Verification items for the finished model (mm, model axes). Round coordinates to 2 decimals unless told otherwise and drop trailing zeros. Write each loop counter-clockwise with the first axis right and the second up, starting at its lowest first coordinate (ties: lowest second). Pieces come first, ordered by that corner, then holes. Notation, with made-up numbers: (3.5, 14.25) - (7.5, 14.25) arc R26 cw to (7.5, 31.25) - close; hole circle Ø5 at (8, 5). An arc over 180 degrees is marked (long way). Answer as a JSON object with one key per item and string values. Group by question number.
1) Section check B-B (z = 143). Enter the section's corners in (x, y).
2) Section check D-D (x = -1). State how many separate pieces and enclosed holes the cut face has, then the cut area to 3 significant figures.
3) Go/stop test with flat-tipped pins: pin 1 Ø4 at (x, z) = (-5.5, 96) entering from -Y; pin 2 Ø6 at (x, y) = (-3, -152) entering from +Z. Record where each tip stops, or that it passes through.
4) Section check C-C (y = -149). Enter the section's corners in (x, z).
5) Thickness scan on line 1 (Z direction, x = 3.5, y = 904); line 2 (Y direction, x = -4.25, z = 289.5); line 3 (Z direction, x = 9, y = 1010). Record the ranges inside material, lowest first.
6) Section check A-A (y = 163). Enter the section's corners in (x, z).
```python
from build123d import *

# Parameters (mm, degrees)
SKETCH1_W           = 2
SKETCH1_H           = 2
SKETCH1_W_2         = 1.6
SKETCH1_H_2         = 1.6
BOSS_EXTRUDE1_DEPTH = 109
SKETCH2_W           = 2
SKETCH2_H           = 2
SKETCH2_W_2         = 1.6
SKETCH2_H_2         = 1.6
BOSS_EXTRUDE2_DEPTH = 34
SKETCH3_W           = 2
SKETCH3_H           = 2
SKETCH3_W_2         = 1.6
SKETCH3_H_2         = 1.6
BOSS_EXTRUDE3_DEPTH = 6
SKETCH7_W           = 2
SKETCH7_H           = 2
SKETCH7_W_2         = 1.54
SKETCH7_H_2         = 1.54
BOSS_EXTRUDE4_DEPTH = 36
BOSS_EXTRUDE5_REACH = 28
SKETCH8_W           = 2
SKETCH8_H           = 2
SKETCH8_W_2         = 1.6
SKETCH8_H_2         = 1.6
SCALE2_SCALE        = 10
BOSS_EXTRUDE6_REACH = 1412
SKETCH9_W           = 20
SKETCH9_H           = 20
SKETCH9_W_2         = 16
SKETCH9_H_2         = 16
SKETCH10_W          = 20
SKETCH10_H          = 20
SKETCH10_W_2        = 16
SKETCH10_H_2        = 16
BOSS_EXTRUDE7_DEPTH = 179.85


with BuildPart() as part:
    # Sketch1 → Boss-Extrude1 (new body)
    with BuildSketch(Plane(origin=(0, 0, 0), x_dir=(1, 0, 0), z_dir=(0, 1, 0))):
        Rectangle(SKETCH1_W, SKETCH1_H)
        Rectangle(SKETCH1_W_2, SKETCH1_H_2, mode=Mode.SUBTRACT)
    boss_extrude1 = extrude(amount=BOSS_EXTRUDE1_DEPTH)

    # Sketch2 → Boss-Extrude2 (add)
    with BuildSketch(Plane.XY.offset(1)):
        with Locations((0, 108)):
            Rectangle(SKETCH2_W, SKETCH2_H)
        with Locations((0, 108)):
            Rectangle(SKETCH2_W_2, SKETCH2_H_2, mode=Mode.SUBTRACT)
    extrude(amount=BOSS_EXTRUDE2_DEPTH)

    # Mirror1: Boss-Extrude1 across plane
    add(boss_extrude1.mirror(Plane.XY.offset(17)))

    # Sketch3 → Boss-Extrude3 (add)
    with BuildSketch(Plane.XY.offset(1)):
        with Locations((0, 1)):
            Rectangle(SKETCH3_W, SKETCH3_H)
        with Locations((0, 1)):
            Rectangle(SKETCH3_W_2, SKETCH3_H_2, mode=Mode.SUBTRACT)
    boss_extrude3 = extrude(amount=BOSS_EXTRUDE3_DEPTH)

    # Sketch7 → Boss-Extrude4 (add)
    with BuildSketch(Plane(origin=(0, 2, 0), x_dir=(1, 0, 0), z_dir=(0, 1, 0))):
        with Locations((0, -8)):
            Rectangle(SKETCH7_W, SKETCH7_H)
        with Locations((0, -8)):
            Rectangle(SKETCH7_W_2, SKETCH7_H_2, mode=Mode.SUBTRACT)
    boss_extrude4 = extrude(amount=-BOSS_EXTRUDE4_DEPTH)

    # Mirror2: Boss-Extrude3, Boss-Extrude4 across plane
    add(boss_extrude3.mirror(Plane.XY.offset(17)))
    add(boss_extrude4.mirror(Plane.XY.offset(17)))

    # Sketch8 → Boss-Extrude5 (add, up to next)
    with BuildSketch(Plane(origin=(0, 0, 25), x_dir=(-1, 0, 0), z_dir=(0, 0, -1)), mode=Mode.PRIVATE) as boss_extrude5_sk1:
        with Locations((0, -33)):
            Rectangle(SKETCH8_W, SKETCH8_H)
        with Locations((0, -33)):
            Rectangle(SKETCH8_W_2, SKETCH8_H_2, mode=Mode.SUBTRACT)
    boss_extrude5_tool1 = extrude(boss_extrude5_sk1.sketch, amount=BOSS_EXTRUDE5_REACH, mode=Mode.PRIVATE) - part.part
    add(boss_extrude5_tool1.solids().sort_by_distance((0, -32.028284, 25))[0])


with BuildPart() as part_1:
    # Scale2: scaled about (0, 0, 0)
    add(part.part.scale(SCALE2_SCALE))

    # Sketch9 → Boss-Extrude6 (add, up to next)
    with BuildSketch(Plane.XZ.offset(-1070), mode=Mode.PRIVATE) as boss_extrude6_sk1:
        with Locations((0, 169.738105544)):
            Rectangle(SKETCH9_W, SKETCH9_H)
        with Locations((0, 169.738105544)):
            Rectangle(SKETCH9_W_2, SKETCH9_H_2, mode=Mode.SUBTRACT)
    boss_extrude6_tool1 = extrude(boss_extrude6_sk1.sketch, amount=BOSS_EXTRUDE6_REACH, mode=Mode.PRIVATE) - part_1.part
    add(boss_extrude6_tool1.solids().sort_by_distance((0, 1070, 179.455263))[0])

    # Sketch10 → Boss-Extrude7 (add)
    with BuildSketch(Plane.XZ.offset(340)):
        with Locations((0, 170)):
            Rectangle(SKETCH10_W, SKETCH10_H)
        with Locations((0, 170)):
            Rectangle(SKETCH10_W_2, SKETCH10_H_2, mode=Mode.SUBTRACT)
    extrude(amount=BOSS_EXTRUDE7_DEPTH)


solid = part_1.part
```
Returned:
{
 "1": {"outline": "(-10, -340) - (10, -340) - (10, -320) - (-10, -320) - close; (-10, 1070) - (10, 1070) - (10, 1090) - (-10, 1090) - close; hole (-8, -338) - (8, -338) - (8, -322) - (-8, -322) - close; hole (-8, 1072) - (8, 1072) - (8, 1088) - (-8, 1088) - close"},
 "2": {"separate pieces": "2", "enclosed holes": "6", "area": "20,800 mm2"},
 "3": {"pin 1": "y = -340", "pin 2": "z = 270"},
 "4": {"outline": "(-10, 70) - (10, 70) - (10, 90) - (-10, 90) - close; (-10, 159.74) - (10, 159.74) - (10, 179.74) - (-10, 179.74) - close; (-10, 250) - (10, 250) - (10, 270) - (-10, 270) - close; hole (-8, 161.74) - (8, 161.74) - (8, 177.74) - (-8, 177.74) - close; hole (-7.7, 72.3) - (7.7, 72.3) - (7.7, 87.7) - (-7.7, 87.7) - close; hole (-7.7, 252.3) - (7.7, 252.3) - (7.7, 267.7) - (-7.7, 267.7) - close"},
 "5": {"line 1": "-10 to -8, 8 to 10, 159.74 to 161.74, 177.74 to 179.74, 330 to 332, 348 to 350", "line 2": "0 to 2, 18 to 20, 1070 to 1072, 1088 to 1090", "line 3": "-10 to 10, 159.74 to 179.74, 330 to 350"},
 "6": {"outline": "(-10, -10) - (10, -10) - (10, 10) - (-10, 10) - close; (-10, 159.74) - (10, 159.74) - (10, 179.74) - (-10, 179.74) - close; (-10, 330) - (10, 330) - (10, 350) - (-10, 350) - close; hole (-8, -8) - (8, -8) - (8, 8) - (-8, 8) - close; hole (-8, 161.74) - (8, 161.74) - (8, 177.74) - (-8, 177.74) - close; hole (-8, 332) - (8, 332) - (8, 348) - (-8, 348) - close"}
}
